Can you work these out from the model? Positions are in its coordinate system, mm. A direction names the side the tool comes from. Round coordinates to 2 decimals unless told otherwise and drop trailing zeros. Loops run counter-clockwise (first coordinate to the right, second up) from the corner with the lowest first, then second, coordinate; pieces in that order, holes last.
```python
from build123d import *

# Parameters (mm, degrees)
EXTRUDE_1_DEPTH     = 20
EXTRUDE_2_DEPTH     = 200
EXTRUDE_3_DEPTH     = 20
SKETCH_5_R          = 2.5
CUT_EXTRUDE_1_DEPTH = 10
CUT_EXTRUDE_START   = -10
SKETCH_6_R          = 2.5
CUT_EXTRUDE_2_DEPTH = 10
CUT_EXTRUDE_3_REACH = 304.324
SKETCH_7_R          = 5


with BuildPart() as part:
    # 草图1 → 凸台-拉伸1 (new body)
    with BuildSketch(Plane(origin=(0, 0, 0), x_dir=(0, 0, -1), z_dir=(1, 0, 0))):
        with BuildLine():
            Line((10, 130), (130, 130))
            Line((130, 130), (130, -10))
            Line((130, -10), (-10, -10))
            Line((-10, -10), (-10, 110))
            ThreePointArc((-10, 110), (-4.142135624, 124.142135624), (10, 130))
        make_face()
        with BuildLine():
            Line((10, 0), (110, 0))
            ThreePointArc((110, 0), (117.071067812, 2.928932188), (120, 10))
            Line((120, 10), (120, 110))
            ThreePointArc((120, 110), (117.071067812, 117.071067812), (110, 120))
            Line((110, 120), (10, 120))
            ThreePointArc((10, 120), (2.928932188, 117.071067812), (0, 110))
            Line((0, 110), (0, 10))
            ThreePointArc((0, 10), (2.928932188, 2.928932188), (10, 0))
        make_face(mode=Mode.SUBTRACT)
    extrude(amount=EXTRUDE_1_DEPTH)

    # 草图2 → 凸台-拉伸2 (add)
    with BuildSketch(Plane(origin=(20, 0, 0), x_dir=(0, 0, -1), z_dir=(1, 0, 0))):
        with BuildLine():
            Line((130, 130), (100, 130))
            Line((100, 130), (100, 125))
            Line((100, 125), (90, 125))
            Line((90, 125), (90, 120))
            Line((90, 120), (107.421459813, 120))
            Line((107.421459813, 120), (110, 120))
            ThreePointArc((110, 120), (117.071067812, 117.071067812), (120, 110))
            Line((120, 110), (120, 10))
            ThreePointArc((120, 10), (117.071067812, 2.928932188), (110, 0))
            Line((110, 0), (10, 0))
            ThreePointArc((10, 0), (2.928932188, 2.928932188), (0, 10))
            Line((0, 10), (-5, 10))
            Line((-5, 10), (-5, 20))
            Line((-5, 20), (-10, 20))
            Line((-10, 20), (-10, 10))
            Line((-10, 10), (-10, -10))
            Line((-10, -10), (130, -10))
            Line((130, -10), (130, 130))
        make_face()
    extrude(amount=EXTRUDE_2_DEPTH)

    # 草图3 → 凸台-拉伸3 (add)
    with BuildSketch(Plane(origin=(220, 0, 0), x_dir=(0, 0, -1), z_dir=(1, 0, 0))):
        with BuildLine():
            Line((130, 130), (10, 130))
            ThreePointArc((10, 130), (-4.142135624, 124.142135624), (-10, 110))
            Line((-10, 110), (-10, -10))
            Line((-10, -10), (130, -10))
            Line((130, -10), (130, 130))
        make_face()
        with BuildLine():
            Line((0, 110), (0, 10))
            ThreePointArc((0, 10), (2.928932188, 2.928932188), (10, 0))
            Line((10, 0), (110, 0))
            ThreePointArc((110, 0), (117.071067812, 2.928932188), (120, 10))
            Line((120, 10), (120, 110))
            ThreePointArc((120, 110), (117.071067812, 117.071067812), (110, 120))
            Line((110, 120), (10, 120))
            ThreePointArc((10, 120), (2.928932188, 117.071067812), (0, 110))
        make_face(mode=Mode.SUBTRACT)
    extrude(amount=EXTRUDE_3_DEPTH)

    # 草图5 → 切除-拉伸1 (cut)
    with BuildSketch(Plane(origin=(240, 0, 0), x_dir=(0, 0, -1), z_dir=(1, 0, 0))):
        with Locations((-5, -5)):
            Circle(SKETCH_5_R)
        with Locations((125, -5)):
            Circle(SKETCH_5_R)
        with Locations((125, 125)):
            Circle(SKETCH_5_R)
    extrude(amount=-CUT_EXTRUDE_1_DEPTH, mode=Mode.SUBTRACT)

    # 草图6 → 切除-拉伸2 (cut)
    with BuildSketch(Plane.ZY.offset(CUT_EXTRUDE_START)):
        with Locations(Location((-125, 125, 0), (0, 0, 180))):
            Circle(SKETCH_6_R)
        with Locations(Location((-125, -5, 0), (0, 0, 180))):
            Circle(SKETCH_6_R)
        with Locations(Location((5, -5, 0), (0, 0, 180))):
            Circle(SKETCH_6_R)
    extrude(amount=CUT_EXTRUDE_2_DEPTH, mode=Mode.SUBTRACT)

    # 草图7 → 切除-拉伸3 (cut, up to next)
    with BuildSketch(Plane.XY.offset(-120), mode=Mode.PRIVATE) as cut_extrude_3_sk1:
        with Locations((120, 60)):
            Circle(SKETCH_7_R)
    cut_extrude_3_tool1 = extrude(cut_extrude_3_sk1.sketch, amount=-CUT_EXTRUDE_3_REACH, mode=Mode.PRIVATE) & part.part
    add(cut_extrude_3_tool1.solids().sort_by_distance((120, 60, -120))[0], mode=Mode.SUBTRACT)


solid = part.part
```
(1) Which directions (+Z, -Z, +X, -X, +Y, -Y) give clear straight access to the entire face, cutting with the end or side of a thin tool? Please do faces 1 (the cylindrical face through (5.07, 122.89, -126.34)), 2 (the flat face through (230, -5, 5)), 3 (the flat face through (119, 15, 5)), 4 (the flat face through (119, 128, -100)), 5 (the flat face through (118, 48, -120)).
(2) For pin 1 (6 mm diameter, centred on y = 125, z = -125, fed in from +X); pin 2 (4 mm diameter, centred on x = 40, z = -86, fed in from +Y); pin 3 (1.5 mm diameter, centred on x = 75, z = 6.5, fed in from +Y); pin 4 (8 mm diameter, centred on x = 113.5, z = -94, fed in from +Y), each with a flat end and sliding along its axis, tell me the tip position at first contact or that it passes through.
(3) If I drill on line 1 (Z direction, x = 4, y = -5); line 2 (Y direction, x = 5.25, z = -125); line 3 (X direction, y = 63.5, z = 2), over which ranges is the centre line in solid material (lowest first)?
(4) Suppose I cut it at A-A (y = 83). Write out the boundary of the cut face in (x, z).
(5) Suppose I cut it at D-D (x = 216). Write out the boundary of the cut face in (y, z).
(6) We'd pull the mould along Z, two halves only. Please class faces 6 (the flat face through (118, 120, -94)), 7 (the flat face through (118, 11, 10)), 8 (the flat face through (118, -10, -59)): released by +Z, released by -Z, zero draft, split by the parting line, or undercut.
(7) Suppose I cut it at C-C (x = 120). Write out the boundary of the cut face in (y, z).
(8) Suppose I cut it at B-B (z = -40.5). Write out the boundary of the cut face in (x, y).
Check result:
1. face 1: -X
1. face 2: +X
1. face 3: +Y
1. face 4: +Z, +Y
1. face 5: +X, -X
2. pin 1: stops at x = 240
2. pin 2: stops at y = 0
2. pin 3: stops at y = 20
2. pin 4: stops at y = 125
3. line 1: z = -130 to -127.5, -122.5 to 2.5, 7.5 to 10
3. line 2: y = -10 to -7.5, -2.5 to 122.5, 127.5 to 130
3. line 3: x = 0 to 20, 220 to 240
4. outline: (0, -130) - (240, -130) - (240, -120) - (0, -120) - close; (0, 0) - (20, 0) - (20, 10) - (0, 10) - close; (220, 0) - (240, 0) - (240, 10) - (220, 10) - close
5. outline: (-10, -130) - (130, -130) - (130, -100) - (125, -100) - (125, -90) - (120, -90) - (120, -110) arc R10 cw to (110, -120) - (10, -120) arc R10 cw to (0, -110) - (0, -10) arc R10 cw to (10, 0) - (10, 5) - (20, 5) - (20, 10) - (-10, 10) - close
6. face 6: undercut
6. face 7: released by +Z
6. face 8: zero draft
7. outline: (-10, -130) - (55, -130) - (55, -120) - (10, -120) arc R10 cw to (0, -110) - (0, -10) arc R10 cw to (10, 0) - (10, 5) - (20, 5) - (20, 10) - (-10, 10) - close; (65, -130) - (130, -130) - (130, -100) - (125, -100) - (125, -90) - (120, -90) - (120, -110) arc R10 cw to (110, -120) - (65, -120) - close
8. outline: (0, -10) - (240, -10) - (240, 0) - (0, 0) - close; (0, 120) - (20, 120) - (20, 130) - (0, 130) - close; (220, 120) - (240, 120) - (240, 130) - (220, 130) - close
